Can you work these out from the drawing? Everything is in mm from the part's minimum corner. A direction names the side the tool comes from. Give positions to 0.01 mm unless a question says otherwise; leave off trailing zeros. Order: outer loops, then holes, each group sorted by start corner. A loop starts at its lowest first (then second) coordinate and runs counter-clockwise, first axis right, second up. Notation, with made-up numbers: M -31,81.25 L 0,81.25 A16 ccw 0,106.25 Z; hole C 36.25,62 d5. An arc over 180 degrees is marked long. Answer in a Markdown table with one row per item. Add a question column.
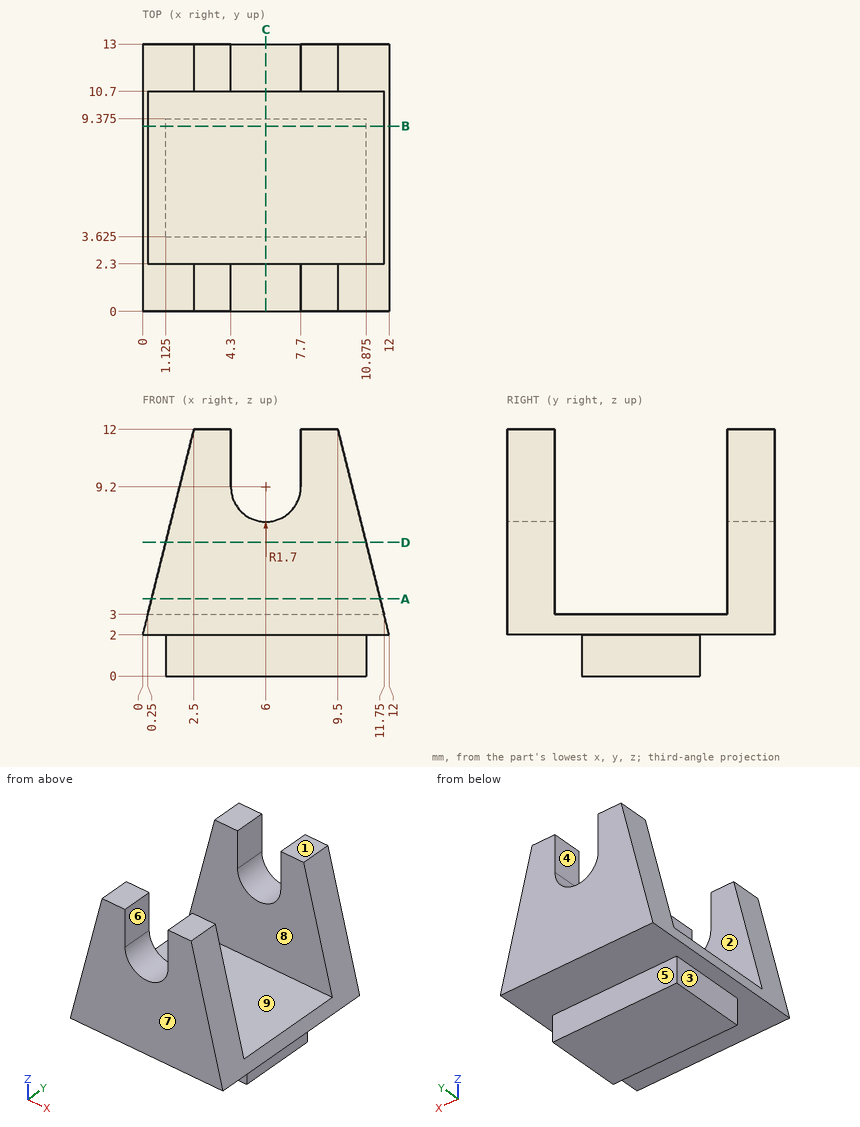
1. For the marked faces 1, 2, 3, 4 and 5, which set-ups out of +Z, -Z, +X, -X, +Y, -Y let a thin tool reach every point of the face, with its end or its side?
2. Will these pins go through, and if not, where does the flat tip stop? P1, Ø1.2, axis at y = 12.5, z = 10, coming from the +X side; P2, Ø1.2, axis at y = 1, z = 11, coming from the +X side; P3, Ø1.5, axis at y = 5, z = 4.5, coming from the -X side; P4, Ø2.5, axis at y = 1.5, z = 10, coming from the -X side.
3. Suppose I cut it at A-A on z = 3.75. List the corners of the cut face in (x, y) for me.
4. Suppose I cut it at B-B on y = 9. List the corners of the cut face in (x, z) for me (3 decimals), plus the area to 4 significant figures.
5. If I drill on line 1 along Y through (x, z) = (4.75, 3.25); line 2 along Z through (x, y) = (8.5, 8.25); line 3 along Z through (x, y) = (10.75, 10.5), over which ranges is the centre line in solid material (lowest first)? Write a range as [from, to].
6. Suppose I cut it at C-C on x = 6. List the corners of the cut face in (y, z) for me (3 decimals), plus the area to 3 significant figures.
7. Suppose I cut it at D-D on z = 6.5. List the corners of the cut face in (x, y) for me (3 decimals).
8. Thinking about a two-plate mould opening in Y: for the marked faces 6, 7, 8 and 9, which applies, pulls with the +Y half, pulls with the -Y half, needs draft (parallel to the pull), parting line crosses it, or undercut?
Findings below:
| question | item | result |
|---|---|---|
| 1 | face 1 | +Z, +X, -X, +Y, -Y |
| 1 | face 2 | +Z, +X, -X |
| 1 | face 3 | -Z, -X, +Y, -Y |
| 1 | face 4 | +Z, +Y, -Y |
| 1 | face 5 | -Z, +X, -X, +Y |
| 2 | P1 | x = 10.15 |
| 2 | P2 | x = 9.9 |
| 2 | P3 | through |
| 2 | P4 | x = 1.69 |
| 3 | outline | M 0.44,0 L 11.56,0 L 11.56,2.3 L 0.44,2.3 Z; M 0.44,10.7 L 11.56,10.7 L 11.56,13 L 0.44,13 Z |
| 4 | outline | M 0,2 L 1.125,2 L 1.125,0 L 10.875,0 L 10.875,2 L 12,2 L 11.75,3 L 0.25,3 Z |
| 4 | area | 31.25 mm2 |
| 5 | line 1 | [0, 2.3], [10.7, 13] |
| 5 | line 2 | [0, 3] |
| 5 | line 3 | [2, 3] |
| 6 | outline | M 0,2 L 3.625,2 L 3.625,0 L 9.375,0 L 9.375,2 L 13,2 L 13,7.5 L 10.7,7.5 L 10.7,3 L 2.3,3 L 2.3,7.5 L 0,7.5 Z |
| 6 | area | 45.2 mm2 |
| 7 | outline | M 1.125,0 L 10.875,0 L 10.875,2.3 L 1.125,2.3 Z; M 1.125,10.7 L 10.875,10.7 L 10.875,13 L 1.125,13 Z |
| 8 | face 6 | needs draft |
| 8 | face 7 | pulls with the -Y half |
| 8 | face 8 | undercut |
| 8 | face 9 | undercut |
